Could you check a few things on this model? Use its own coordinates, in mm. A direction names the side the tool comes from. Round coordinates to 2 decimals unless told otherwise and drop trailing zeros. Loops run counter-clockwise (first coordinate to the right, second up) from the corner with the lowest first, then second, coordinate; pieces in that order, holes last. Notation, with made-up numbers: M -12,-35.5 L 40,-35.5 A22 cw 40,1.5 Z; hole C 33,9 d7. An arc over 180 degrees is marked long. One line per item, written item: value. Start each with the question number.
Q1. Imagine slicing it at D-D (x = 2.5). Please give me the cut outline in (y, z).
Q2. Imagine slicing it at A-A (x = 0). Please give me the cut outline in (y, z).
Q3. Imagine slicing it at C-C (z = 24). Please give me the cut outline in (x, y).
Q4. Which directions (+Z, -Z, +X, -X, +Y, -Y) give clear straight access to the entire face, cutting with the end or side of a thin tool? Please do faces 1 (the face through (-2.17, -9.76, 29.74)), 2 (the face through (0, 5.196, 9)), 3 (the face through (0.78, -5.95, 14.3)).
Q5. I'm going to push flat-ended pins straight in: pin 1 Ø4 at (y, z) = (4, 26.5) entering from +X; pin 2 Ø4 at (y, z) = (1, 21.5) entering from +X; pin 3 Ø4 at (x, z) = (-0.5, 24) entering from -Y. Where does each tip first touch, or does it pass through?
Q6. Please list where these lines run through material, in increasing order: line 1 along Z through (x, y) = (6, -6.5); line 2 along Y through (x, z) = (-0.25, 23.5); line 3 along X through (y, z) = (-3, 20).
Q7. Imagine slicing it at B-B (y = 0). Please give me the cut outline in (x, z).
from build123d import *

# Parameters (mm, degrees)
SKETCH1_R           = 6
BOSS_EXTRUDE1_DEPTH = 29
CUT_EXTRUDE1_DEPTH  = 19
SKETCH3_R           = 10
BOSS_EXTRUDE2_DEPTH = 1.5


with BuildPart() as part:
    # Sketch1 → Boss-Extrude1 (new body)
    with BuildSketch(Plane.XY):
        with Locations(Location((0, 0, 0), (0, 0, 180))):
            Circle(SKETCH1_R)
    extrude(amount=BOSS_EXTRUDE1_DEPTH)

    # Sketch2 → Cut-Extrude1 (cut)
    with BuildSketch(Plane(origin=(0, 0, 0), x_dir=(-1, 0, 0), z_dir=(0, 0, -1))):
        Polygon((-41.730042052, 5.196152423), (-3, 5.196152423), (3, 5.196152423), (41.730042052, 5.196152423), (41.730042052, 82.656236526), (-41.730042052, 82.656236526), align=None)
    extrude(amount=-CUT_EXTRUDE1_DEPTH, mode=Mode.SUBTRACT)

    # Sketch3 → Boss-Extrude2 (add)
    with BuildSketch(Plane.XY.offset(29)):
        Circle(SKETCH3_R)
    extrude(amount=BOSS_EXTRUDE2_DEPTH)


solid = part.part
Report:
1. outline: M -9.68,29 L -5.45,29 L -5.45,0 L 5.2,0 L 5.2,19 L 5.45,19 L 5.45,29 L 9.68,29 L 9.68,30.5 L -9.68,30.5 Z
2. outline: M -10,29 L -6,29 L -6,0 L 5.2,0 L 5.2,19 L 6,19 L 6,29 L 10,29 L 10,30.5 L -10,30.5 Z
3. outline: C 0,0 d12
4. face 1: +Z, -Z
4. face 2: -Z, +X, -X, +Y
4. face 3: -Z
5. pin 1: stops at x = 5.66
5. pin 2: stops at x = 6
5. pin 3: stops at y = -6
6. line 1: z = 29 to 30.5
6. line 2: y = -5.99 to 5.99
6. line 3: x = -5.2 to 5.2
7. outline: M -10,29 L -6,29 L -6,0 L 6,0 L 6,29 L 10,29 L 10,30.5 L -10,30.5 Z
